from build123d import *

# Parameters (mm, degrees)
F0_W      = 177.8
F0_H      = 34.925
F1_DEPTH  = 76.2
F2_W      = 82.55
F2_H      = 76.2
F3_DEPTH  = 88.9
F5_DEPTH  = 76.201
F6_R      = 19.05
F7_DEPTH  = 12.7
F8_R      = 12.7
F9_DEPTH  = 34.926
F10_R     = 19.05
F11_DEPTH = 12.7
F12_R     = 12.7
F13_DEPTH = 76.201


with BuildPart() as f1:
    # F0 (on Front) → F1 (new body)
    with BuildSketch(Plane.XZ):
        with Locations((88.9, 17.4625)):
            Rectangle(F0_W, F0_H)
    extrude(amount=F1_DEPTH)

    # F2 (on face) → F3 (join)
    with BuildSketch(Plane.XY.offset(34.925)):
        with Locations((41.275, -38.1)):
            Rectangle(F2_W, F2_H)
    extrude(amount=F3_DEPTH)

    # F4 (on face) → F5 (cut, through all)
    with BuildSketch(Plane.XZ.offset(76.2)):
        with BuildLine():
            ThreePointArc((0, 76.2), (41.275, 117.475), (82.55, 76.2))
            Line((82.55, 76.2), (82.55, 123.825))
            Line((82.55, 123.825), (0, 123.825))
            Line((0, 123.825), (0, 76.2))
        make_face()
    extrude(amount=-F5_DEPTH, mode=Mode.SUBTRACT)

    # F6 (on face) → F7 (cut)
    with BuildSketch(Plane.XY.offset(34.925)):
        with Locations((139.7, -38.1)):
            Circle(F6_R)
    extrude(amount=-F7_DEPTH, mode=Mode.SUBTRACT)

    # F8 (on face) → F9 (cut, through all)
    with BuildSketch(Plane.XY.offset(34.925)):
        with Locations((139.7, -38.1)):
            Circle(F8_R)
    extrude(amount=-F9_DEPTH, mode=Mode.SUBTRACT)

    # F10 (on face) → F11 (cut)
    with BuildSketch(Plane.XZ.offset(76.2)):
        with Locations((41.275, 76.2)):
            Circle(F10_R)
    extrude(amount=-F11_DEPTH, mode=Mode.SUBTRACT)

    # F12 (on face) → F13 (cut, through all)
    with BuildSketch(Plane.XZ.offset(76.2)):
        with Locations((41.275, 76.2)):
            Circle(F12_R)
    extrude(amount=-F13_DEPTH, mode=Mode.SUBTRACT)


solid = f1.part
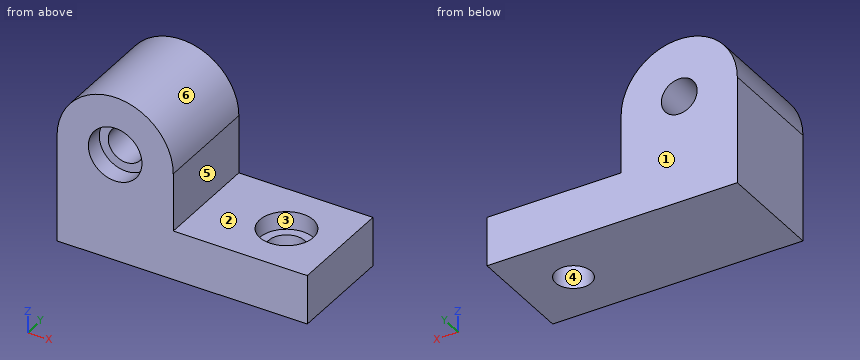
Verification items for the finished model (mm, model axes). Face numbers are marked on the shaded views. A direction names the side the tool comes from. Coordinates: 2 decimals unless noted, no trailing zeros. Write each loop counter-clockwise with the first axis right and the second up, starting at its lowest first coordinate (ties: lowest second). Pieces come first, ordered by that corner, then holes. Notation, with made-up numbers: M -28,34 L -4,34 A21 cw -4,64 Z; hole C 49.25,28.25 d2. An arc over 180 degrees is marked long. Use CSV: the item, a comma, the result in double quotes.
Q1. Thickness scan on line 1 along X through (y, z) = (-38, 27); line 2 along Y through (x, z) = (139, 30); line 3 along X through (y, z) = (-14, 76). Record the ranges inside material, lowest first. Write a range as [from, to].
Computed values:
line 1,"[0, 120.65], [158.75, 177.8]"
line 2,"[-76.2, -57.14], [-19.06, 0]"
line 3,"[0, 28.58], [53.97, 82.55]"
Q2. Section check B-B, the plane x = 139.7. Enter the section's corners in (y, z) (3 decimals).
Computed values:
outline,"M -76.2,0 L -50.8,0 L -50.8,22.225 L -57.15,22.225 L -57.15,34.925 L -76.2,34.925 Z; M -25.4,0 L 0,0 L 0,34.925 L -19.05,34.925 L -19.05,22.225 L -25.4,22.225 Z"
Q3. Section check C-C, the plane y = -68.5. Enter the section's corners in (x, z) (3 decimals).
Computed values:
outline,"M 0,0 L 177.8,0 L 177.8,34.925 L 82.55,34.925 L 82.55,76.2 A41.275 ccw 0,76.2 Z; hole C 41.275,76.2 d38.1"
Q4. Go/stop test with flat-tipped pins: P1, Ø20.5, axis at x = 139.7, y = -38.1, coming from the -Z side; P2, Ø19, axis at x = 37, z = 84, coming from the -Y side; P3, Ø23, axis at x = 130.5, y = -37, coming from the +Z side (3 decimals); P4, Ø1.5, axis at y = -60.5, z = 79, coming from the -X side. Record where each tip stops, or that it passes through.
Computed values:
P1,"through"
P2,"y = -63.5"
P3,"z = 34.925"
P4,"x = 0.05"
Q5. Section check D-D, the plane z = 74. Enter the section's corners in (x, y), and give its area (3 significant figures).
Computed values:
outline,"M 0,-76.2 L 22.35,-76.2 L 22.35,-63.5 L 28.77,-63.5 L 28.77,0 L 0,0 Z; M 53.78,-63.5 L 60.2,-63.5 L 60.2,-76.2 L 82.55,-76.2 L 82.55,0 L 53.78,0 Z"
area,"4,220 mm²"
Q6. Mould release check, pull along Y, two halves, no side actions. Record for the marked faces 1, 2, 3 and 4: pulls with the +Y half, pulls with the -Y half, needs draft (parallel to the pull), parting line crosses it, or undercut.
Computed values:
face 1,"pulls with the +Y half"
face 2,"needs draft"
face 3,"undercut"
face 4,"undercut"
Q7. Section check A-A, the plane y = -38.1. Enter the section's corners in (x, z) (3 decimals), and give its area (3 significant figures).
Computed values:
outline,"M 0,0 L 127,0 L 127,22.225 L 120.65,22.225 L 120.65,34.925 L 82.55,34.925 L 82.55,76.2 A41.275 ccw 0,76.2 Z; M 152.4,0 L 177.8,0 L 177.8,34.925 L 158.75,34.925 L 158.75,22.225 L 152.4,22.225 Z; hole C 41.275,76.2 d25.4"
area,"10,700 mm²"
Q8. Set-up check for the marked faces 5 and 6: record each of +Z, -Z, +X, -X, +Y, -Y from which the full face is reachable in a straight line by a thin tool's end or side.
Computed values:
face 5,"+Z, +X, +Y, -Y"
face 6,"+Z, +Y, -Y"
